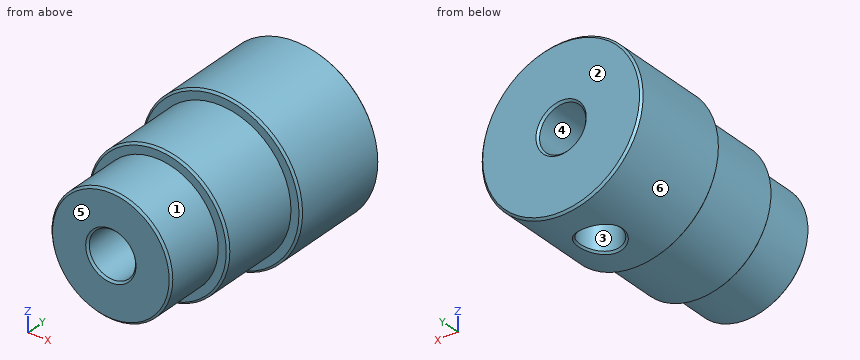
Autodesk Inventor part; units mm, degrees
ref_plane "YZ Plane" through (0, 0, 0) normal (1, 0, 0) x (0, 1, 0)
ref_plane "XZ Plane" through (0, 0, 0) normal (0, 1, 0) x (-1, 0, 0)
ref_plane "XY Plane" through (0, 0, 0) normal (0, 0, 1) x (1, 0, 0)
sketch "Skizze1" plane through (0, 0, 0) normal (0, 0, 1) x (1, 0, 0)
  line L0 (0, 5) -> (4, 5)
  line L1 (4, 5) -> (4, 0)
  line L2 (4, 0) -> (3, 0)
  line L3 (3, 0) -> (3, -7)
  line L4 (3, -7) -> (0, -7)
  line L5 (0, -7) -> (0, 5)
  line L6 (3.5, 0) -> (3.5, -4)
  line L7 (3.5, -4) -> (3, -4)
  point P0 (0, 0)
  dimension "d0" = 6
  dimension "d1" = 7
  dimension "d2" = 8
  dimension "d3" = 5
  dimension "d31" = 7
  dimension "d32" = 4
revolve "Umdrehung1" add sketch "Skizze1" angle 360 about axis through (0, -7, 0) along (0, 1, 0)
chamfer "Fase1" distance 0.1 angle 45 4 edges at (-4, 5, 0) (-3, -7, 0) (-4, 0, 0) (-3.5, -4, 0)
hole "Bohrung1" at (0, 5, 0) direction (0, -1, 0) diameter 2.3 end through all both
chamfer "Fase2" distance 0.1 angle 45 2 edges at (0, -7, -1.15) (0, 5, -1.15)
sketch "Skizze2" plane through (0, 0, 0) normal (0, 0, 1) x (1, 0, 0)
  circle A0 centre (0, 2.5) radius 1
  line L0 (1.25, 5) -> (-1.25, 5)
  line L1 (0, 7.4) -> (0, -9.4)
  point P0 (0, 0)
  dimension "d20" = 2
  dimension "d21" = 2.5
extrude "Extrusion1" cut sketch "Skizze2" against normal blind 10
chamfer "Fase3" distance 0.1 angle 45 1 edges at (-1, 2.5012, -3.873)
thread "Gewinde1"
properties part number "nabe" material "Aluminium 6061"
The listing builds one solid part. Answer for the finished solid, in the listing's coordinates (mm). Face numbers are marked on the shaded views. A direction names the side the tool comes from. Coordinates: 2 decimals unless noted, no trailing zeros. Order: outer loops, then holes, each group sorted by start corner. A loop starts at its lowest first (then second) coordinate and runs counter-clockwise, first axis right, second up. Notation, with made-up numbers: (89, 48.25) -> (124, 48.25) arc R23 cw to (124, 84.25) -> close; hole circle Ø1 at (84, 19). An arc over 180 degrees is marked (long way). Answer in a Markdown table with one row per item. Add a question column.
Item 1: Find the intervals of material crossed by L1, parallel to Z at x = 0, y = -3.5; L2, parallel to Z at x = 0, y = 0.5; L3, parallel to Z at x = 0, y = 2, in increasing order. Write a range as from..to.
Item 2: Find section C-C (x = -0.5). State how many separate pieces and enclosed holes the cut face has, then the cut area to 3 significant figures.
Item 3: Each of these flat-tipped pins is pushed along its axis until it touches: P1, Ø1.5, axis at y = -2, z = 0, coming from the -X side; P2, Ø1.2, axis at x = 0, y = 2.5, coming from the -Z side; P3, Ø3, axis at y = -4, z = 2, coming from the +X side. Where does it stop, or does it pass through?
Item 4: Find section D-D (y = -6). Write down the section's boundary in (x, z).
Item 5: Determine the mould class of the marked faces 4, 5 and 6 for opening direction X: +X half, -X half, draft (parallel to the pull), parting line (faces both ways), or undercut.
Item 6: Find section A-A (z = 0). Write down the section's boundary in (x, y).
Item 7: Find section B-B (y = -3). Write down the section's boundary in (x, z).
Item 8: Which of the six approach directions +Z, -Z, +X, -X, +Y, -Y give full straight-line access (tool end or side, diameter ignored) to the marked faces 1, 2 and 3?
Result set:
| question | item | result |
|---|---|---|
| 1 | L1 | z = -3.5..-1.15, 1.15..3.5 |
| 1 | L2 | z = -4..-1.15, 1.15..4 |
| 1 | L3 | z = 1.15..4 |
| 2 | separate pieces | 3 |
| 2 | enclosed holes | 0 |
| 2 | area | 55.1 mm² |
| 3 | P1 | stops at x = -3.5 |
| 3 | P2 | stops at z = 0.98 |
| 3 | P3 | stops at x = 3.46 |
| 4 | outline | circle Ø6 at (0, 0); hole circle Ø2.3 at (0, 0) |
| 5 | face 4 | undercut |
| 5 | face 5 | draft |
| 5 | face 6 | parting line |
| 6 | outline | (-4, 0.1) -> (-3.9, 0) -> (-3.5, 0) -> (-3.5, -3.9) -> (-3.4, -4) -> (-3, -4) -> (-3, -6.9) -> (-2.9, -7) -> (-1.25, -7) -> (-1.15, -6.9) -> (-1.15, 4.9) -> (-1.25, 5) -> (-3.9, 5) -> (-4, 4.9) -> close; (1.15, -6.9) -> (1.25, -7) -> (2.9, -7) -> (3, -6.9) -> (3, -4) -> (3.4, -4) -> (3.5, -3.9) -> (3.5, 0) -> (3.9, 0) -> (4, 0.1) -> (4, 4.9) -> (3.9, 5) -> (1.25, 5) -> (1.15, 4.9) -> close |
| 7 | outline | circle Ø7 at (0, 0); hole circle Ø2.3 at (0, 0) |
| 8 | face 1 | -Y |
| 8 | face 2 | +Z, -Z, +X, -X, +Y |
| 8 | face 3 | -Z |
